Geometry: final body of the model. Coordinates: model frame, mm. Face numbers are marked on the shaded views. A direction names the side the tool comes from. Give positions to 0.01 mm unless a question says otherwise; leave off trailing zeros. Write each loop counter-clockwise with the first axis right and the second up, starting at its lowest first coordinate (ties: lowest second). Pieces come first, ordered by that corner, then holes. Notation, with made-up numbers: (8.25, 75.25) -> (40.25, 75.25) arc R22 ccw to (40.25, 100.25) -> close; hole circle Ø2 at (9.25, 22). An arc over 180 degrees is marked (long way). Answer as a JSON object with one key per item and string values.
from build123d import *

# Parameters (mm, degrees)
EXTRUDE_1_DEPTH     = 60
SKETCH_2_W          = 87
SKETCH_2_H          = 23
EXTRUDE_2_DEPTH     = 2
SKETCH_3_R          = 1.5
CUT_EXTRUDE_1_DEPTH = 2
SKETCH_4_R          = 1.5
CUT_EXTRUDE_2_DEPTH = 5
SKETCH_5_R          = 4
CUT_EXTRUDE_3_DEPTH = 3
CHAMFER_1_SIZE      = 1
CHAMFER_2_SIZE      = 5


with BuildPart() as part:
    # Эскиз1 → Бобышка-Вытянуть1 (new body)
    with BuildSketch(Plane.XY):
        Polygon((30.5, 0), (38.5, 8), (-38.5, 8), (-30.5, 0), (-43.5, 0), (-43.5, 13), (43.5, 13), (43.5, 0), align=None)
    extrude(amount=EXTRUDE_1_DEPTH)

    # Эскиз2 → Бобышка-Вытянуть2 (add)
    with BuildSketch(Plane.XY.offset(60)):
        with Locations((0, 11.5)):
            Rectangle(SKETCH_2_W, SKETCH_2_H)
    extrude(amount=EXTRUDE_2_DEPTH)

    # Эскиз3 → Вырез-Вытянуть1 (cut)
    with BuildSketch(Plane.XY.offset(62)):
        with Locations((-35, 19)):
            Circle(SKETCH_3_R)
        with Locations(Location((35, 19, 0), (0, 0, 180))):
            Circle(SKETCH_3_R)
    extrude(amount=-CUT_EXTRUDE_1_DEPTH, mode=Mode.SUBTRACT)

    # Эскиз4 → Вырез-Вытянуть2 (cut)
    with BuildSketch(Plane.XZ.offset(-8)):
        with Locations((0, 15)):
            Circle(SKETCH_4_R)
    extrude(amount=-CUT_EXTRUDE_2_DEPTH, mode=Mode.SUBTRACT)

    # Эскиз5 → Вырез-Вытянуть3 (cut)
    with BuildSketch(Plane.XZ.offset(-8)):
        with Locations((0, 15)):
            Circle(SKETCH_5_R)
    extrude(amount=-CUT_EXTRUDE_3_DEPTH, mode=Mode.SUBTRACT)

    # Фаска1
    chamfer_1_edges = [part.edges().sort_by_distance(p)[0] for p in [
        (0, 8, 0),
        (-34.5, 4, 0),
        (34.5, 4, 0),
    ]]
    chamfer(chamfer_1_edges, length=CHAMFER_1_SIZE)

    # Фаска2
    chamfer_2_edges = [part.edges().sort_by_distance(p)[0] for p in [
        (43.5, 0, 31),
        (-43.5, 0, 31),
        (-43.5, 23, 61),
        (43.5, 23, 61),
    ]]
    chamfer(chamfer_2_edges, length=CHAMFER_2_SIZE)


solid = part.part
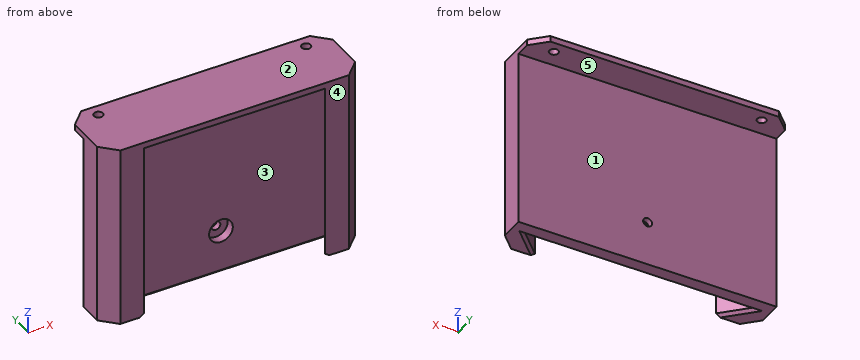
Q1. Material intervals for L1, parallel to Z at x = 0, y = 9.5; L2, parallel to Z at x = 0, y = 11.7; L3, parallel to Y at x = 35, z = 61.1, sorted ascending. Write a range as from..to.
Values:
{"L1": "0..11, 19..62", "L2": "0..13.5, 16.5..62", "L3": "0..17.5, 20.5..23"}
Q2. Set-up query: the marked faces 1 and 2. Return all of +Z, -Z, +X, -X, +Y, -Y with unobstructed straight access to the full face (end or side cutting, diameter ignored); none if empty.
Values:
{"face 1": "-Z, +X, -X, +Y", "face 2": "+Z, +X, -X, +Y, -Y"}
Q3. Mould query, pull axis Y, two halves, no side actions, for the marked faces 3, 4 and 5. Classes: pulls with the +Y half, pulls with the -Y half, needs draft (parallel to the pull), parting line crosses it, or undercut.
Values:
{"face 3": "undercut", "face 4": "pulls with the -Y half", "face 5": "needs draft"}
Q4. Cut plane A-A (x = 0). Return the cut outline in (y, z).
Values:
{"outline": "(0, 60) -> (8, 60) -> (8, 19) -> (11, 19) -> (11, 16.5) -> (13, 16.5) -> (13, 60) -> (23, 60) -> (23, 62) -> (0, 62) -> close; (8, 1) -> (9, 0) -> (13, 0) -> (13, 13.5) -> (11, 13.5) -> (11, 11) -> (8, 11) -> close"}
Q5. Cut plane D-D (x = 10). Return the cut outline in (y, z).
Values:
{"outline": "(0, 60) -> (8, 60) -> (8, 1) -> (9, 0) -> (13, 0) -> (13, 60) -> (23, 60) -> (23, 62) -> (0, 62) -> close"}
Q6. First-contact query: P1, Ø4, axis at x = 23.5, z = 13.5, coming from the +Y side; P2, Ø12, axis at x = -21.5, z = 31.5, coming from the -Y side; P3, Ø5, axis at x = 0, z = 15, coming from the -Y side. Flat tips, straight axial feed; report the tip coordinate or a pass-through.
Values:
{"P1": "y = 13", "P2": "y = 8", "P3": "y = 11"}
Q7. Cut plane C-C (z = 15). Return the cut outline in (x, y).
Values:
{"outline": "(-43.5, 5) -> (-38.5, 0) -> (-30.5, 0) -> (-38.5, 8) -> (-4, 8) -> (-4, 11) -> (-1.5, 11) -> (-1.5, 13) -> (-43.5, 13) -> close; (1.5, 11) -> (4, 11) -> (4, 8) -> (38.5, 8) -> (30.5, 0) -> (38.5, 0) -> (43.5, 5) -> (43.5, 13) -> (1.5, 13) -> close"}
Q8. Cut plane B-B (y = 19). Return the cut outline in (x, z), and give its area (3 significant figures).
Values:
{"outline": "(-42.5, 60) -> (-36.5, 60) -> (-36.5, 62) -> (-42.5, 62) -> close; (-33.5, 60) -> (33.5, 60) -> (33.5, 62) -> (-33.5, 62) -> close; (36.5, 60) -> (42.5, 60) -> (42.5, 62) -> (36.5, 62) -> close", "area": "158 mm²"}
